Verification items for the finished model (mm, model axes). Face numbers are marked on the shaded views. A direction names the side the tool comes from. Coordinates: 2 decimals unless noted, no trailing zeros. Order: outer loops, then holes, each group sorted by start corner. A loop starts at its lowest first (then second) coordinate and runs counter-clockwise, first axis right, second up. Notation, with made-up numbers: M 1.5,88 L 17.5,88 A25 cw 17.5,124 Z; hole C 31.5,52 d5. An arc over 180 degrees is marked long. Answer as a JSON object with one key per item and string values. Group by question number.
(1) Gauge pin test, flat ends, axial feed: pin 1 Ø16.5 at (x, y) = (-38, -35) entering from -Z; pin 2 Ø8 at (y, z) = (-47.5, -2) entering from +X; pin 3 Ø2.5 at (x, y) = (-16.5, -24.5) entering from -Z; pin 4 Ø1.5 at (y, z) = (-52, -10) entering from -X. Record the tip position at first contact, or that the pin passes through.
(2) Access from +Z, -Z, +X, -X, +Y, -Y to the whole of each face (thin tool, end or side, straight path). Record for the marked faces 1, 2, 3 and 4.
(3) Material ranges on line 1 (Y direction, x = -45.5, z = -9.5); line 2 (Z direction, x = -47.5, y = -49.5); line 3 (X direction, y = -26, z = -11), recorded low to high.
(4) Mould release check, pull along X, two halves, no side actions. Record for the marked faces 5, 6 and 7: released by +X, released by -X, zero draft, split by the parting line, or undercut.
(5) Cross-section at D-D (y = -25.5). Enter the section's corners in (x, z).
(6) Cross-section at A-A (z = -6). Enter the section's corners in (x, y).
(7) Cross-section at C-C (y = -51). Enter the section's corners in (x, z), plus the area to 3 significant figures.
(8) Cross-section at B-B (x = -17). Enter the section's corners in (y, z), plus the area to 3 significant figures.
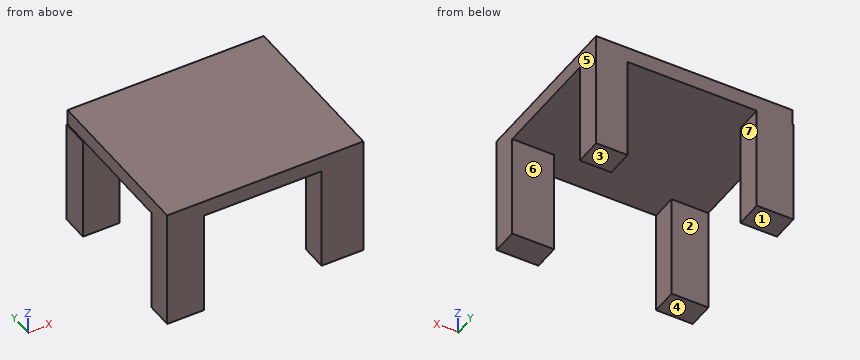
from build123d import *

# Parameters (mm, degrees)
F0_W     = 38.2699640468
F0_H     = 32.5195547193
F1_DEPTH = 3.048
F2_W     = 6.1469888315
F2_H     = 20.1264321804
F2_W_2   = 7.1384422481
F2_H_2   = 20.5230116844
F3_DEPTH = 5.334
F4_W     = 7.1802772582
F4_H     = 23.4715147685
F4_W_2   = 8.1633431837
F5_DEPTH = 5.08


with BuildPart() as f1:
    # F0 (on Top) → F1 (new body)
    with BuildSketch(Plane.XY):
        with Locations((-32.6186991297, -38.7656884268)):
            Rectangle(F0_W, F0_H)
    extrude(amount=F1_DEPTH)

    # F2 (on face) → F3 (join)
    with BuildSketch(Plane(origin=(0, -22.5059110671, 0), x_dir=(-1, 0, 0), z_dir=(0, 1, 0))):
        with Locations((16.557211522, -10.0632160902)):
            Rectangle(F2_W, F2_H)
        with Locations((48.382749781, -10.2615058422)):
            Rectangle(F2_W_2, F2_H_2)
    extrude(amount=-F3_DEPTH)

    # F4 (on face) → F5 (join)
    with BuildSketch(Plane.XZ.offset(55.0254657865)):
        with Locations((-48.163542524, -8.6877573842)):
            Rectangle(F4_W, F4_H)
        with Locations((-17.5653886981, -8.6877573842)):
            Rectangle(F4_W_2, F4_H)
    extrude(amount=-F5_DEPTH)


solid = f1.part
Taken from the geometry:
{
 "1": {"pin 1": "stops at z = 0", "pin 2": "stops at x = -13.48", "pin 3": "stops at z = -20.13", "pin 4": "stops at x = -51.75"},
 "2": {"face 1": "-Z, +X, -X, +Y, -Y", "face 2": "-Z, +X, -X", "face 3": "-Z, +X, +Y", "face 4": "-Z, +X, -X, -Y"},
 "3": {"line 1": "y = -55.03 to -49.95, -27.84 to -22.51", "line 2": "z = 0 to 3.05", "line 3": "x = -51.95 to -44.81, -19.63 to -13.48"},
 "4": {"face 5": "released by +X", "face 6": "zero draft", "face 7": "undercut"},
 "5": {"outline": "M -51.95,-20.52 L -44.81,-20.52 L -44.81,0 L -19.63,0 L -19.63,-20.13 L -13.48,-20.13 L -13.48,3.05 L -51.75,3.05 L -51.75,0 L -51.95,0 Z"},
 "6": {"outline": "M -51.95,-27.84 L -44.81,-27.84 L -44.81,-22.51 L -51.95,-22.51 Z; M -51.75,-55.03 L -44.57,-55.03 L -44.57,-49.95 L -51.75,-49.95 Z; M -21.65,-55.03 L -13.48,-55.03 L -13.48,-49.95 L -21.65,-49.95 Z; M -19.63,-27.84 L -13.48,-27.84 L -13.48,-22.51 L -19.63,-22.51 Z"},
 "7": {"outline": "M -51.75,-20.42 L -44.57,-20.42 L -44.57,0 L -21.65,0 L -21.65,-20.42 L -13.48,-20.42 L -13.48,3.05 L -51.75,3.05 Z", "area": "430 mm²"},
 "8": {"outline": "M -55.03,-20.42 L -49.95,-20.42 L -49.95,0 L -27.84,0 L -27.84,-20.13 L -22.51,-20.13 L -22.51,3.05 L -55.03,3.05 Z", "area": "310 mm²"}
}
